Autodesk Inventor part; units mm, degrees
ref_plane "YZ Plane" through (0, 0, 0) normal (1, 0, 0) x (0, 1, 0)
ref_plane "XZ Plane" through (0, 0, 0) normal (0, 1, 0) x (-1, 0, 0)
ref_plane "XY Plane" through (0, 0, 0) normal (0, 0, 1) x (1, 0, 0)
sketch "Sketch1" plane through (0, 0, 0) normal (0, 0, 1) x (1, 0, 0)
  line L0 (37.0001, -37.0002) -> (-37.0001, -37.0002)
  line L1 (-37.0001, -37.0002) -> (-37.0001, 37.0002)
  line L2 (-37.0001, 37.0002) -> (37.0001, 37.0002)
  line L3 (37.0001, 37.0002) -> (37.0001, -37.0002)
  line L4 (69.0001, -5.0002) -> (-5.0001, 69.0002) construction
  circle A0 centre (32, 32) radius 1.5
  circle A1 centre (32, -32) radius 1.5
  circle A2 centre (-32, 32) radius 1.5
  line L5 (5.0001, -69.0002) -> (-69.0001, 5.0002) construction
  circle A3 centre (-32, -32) radius 1.5
  line L6 (37.0001, -101.0002) -> (-37.0001, -26.9998) construction
  line L7 (5.0001, -69.0002) -> (-69.0001, 5.0002) construction
extrude "Extrusion1" add sketch "Sketch1" along normal blind 22
fillet "Fillet1" radius 5 4 edges at (-37.0001, 37.0002, 11) (37.0001, 37.0002, 11) (37.0001, -37.0002, 11) (-37.0001, -37.0002, 11)
sketch "Sketch2" plane through (0, 0, 0) normal (0, 0, -1) x (-1, 0, 0)
  point P0 (0, 0)
sketch "Sketch4" plane through (0, 0, 22) normal (0, 0, 1) x (1, 0, 0)
  point P0 (0, 0)
sketch "Sketch5" plane through (0, 0, 22) normal (0, 0, 1) x (1, 0, 0)
  line L0 (-37.0001, 32.0002) -> (-37.0001, -32.0002)
  line L1 (-26.9999, 37.0018) -> (-37.0001, 37.0018)
  line L2 (-37.0001, 37.0018) -> (-37.0001, 26.9982)
  line L3 (-37.0001, 26.9982) -> (-26.9999, 26.9982)
  line L4 (-26.9999, 26.9982) -> (-26.9999, 37.0018)
  circle A0 centre (-32, 32) radius 1.5
  line L5 (-26.9999, 37.0018) -> (-37.0001, 26.9982) construction
  line L6 (-37.0001, 37.0018) -> (-26.9999, 26.9982) construction
  line L7 (37.0001, 37.0018) -> (26.9999, 37.0018)
  line L8 (26.9999, 37.0018) -> (26.9999, 26.9982)
  line L9 (26.9999, 26.9982) -> (37.0001, 26.9982)
  line L10 (37.0001, 26.9982) -> (37.0001, 37.0018)
  line L11 (37.0001, 37.0018) -> (26.9999, 26.9982) construction
  line L12 (26.9999, 37.0018) -> (37.0001, 26.9982) construction
  line L13 (-26.9999, -26.9982) -> (-37.0001, -26.9982)
  line L14 (-37.0001, -26.9982) -> (-37.0001, -37.0018)
  line L15 (-37.0001, -37.0018) -> (-26.9999, -37.0018)
  line L16 (-26.9999, -37.0018) -> (-26.9999, -26.9982)
  line L17 (-26.9999, -26.9982) -> (-37.0001, -37.0018) construction
  line L18 (-37.0001, -26.9982) -> (-26.9999, -37.0018) construction
  line L19 (37.0001, -26.9982) -> (26.9999, -37.0018) construction
  line L20 (37.0001, -37.0018) -> (37.0001, -26.9982)
  line L21 (26.9999, -37.0018) -> (37.0001, -37.0018)
  line L22 (26.9999, -26.9982) -> (26.9999, -37.0018)
  line L23 (37.0001, -26.9982) -> (26.9999, -26.9982)
  line L24 (26.9999, -26.9982) -> (37.0001, -37.0018) construction
  point P0 (0, 0)
extrude "Extrusion2" cut sketch "Sketch5" against normal blind 5 contours L2 L1 L4 L3 L0 | L13 L16 L15 L14 L0 | A0 | L10 L9 L8 L7 | L21 L22 L23 L20
fillet "Fillet2" radius 5 4 edges at (-26.9999, 26.9982, 19.5) (26.9999, 26.9982, 19.5) (-26.9999, -26.9982, 19.5) (26.9999, -26.9982, 19.5)
sketch "Sketch6" plane through (0, 0, 22) normal (0, 0, 1) x (1, 0, 0)
  line L0 (96.2626, 67.9332) -> (202.4541, 67.9332) construction
  line L1 (202.4541, 67.9332) -> (202.4541, -70.892) construction
  line L2 (202.4541, -70.892) -> (96.2626, -70.892) construction
  line L3 (96.2626, -70.892) -> (96.2626, 67.9332) construction
  point P0 (0, 0)
decal "Decal3"
properties part number "RTK-F9P-Sirius_rover"
The listing builds one solid part. Answer for the finished solid, in the listing's coordinates (mm). A direction names the side the tool comes from. Give positions to 0.01 mm unless a question says otherwise; leave off trailing zeros. Write each loop counter-clockwise with the first axis right and the second up, starting at its lowest first coordinate (ties: lowest second). Pieces come first, ordered by that corner, then holes.
Item 1: Section A-A, the plane z = 20 is taken. Write down the section's boundary in (x, y), plus the area to 3 significant figures.
Item 2: Determine the mould class of faces 1 (the cylindrical face through (-35, 36, 9)), 2 (the flat face through (-33.2, 33.2, 17)), 3 (the cylindrical face through (-33.2, 32.9, 8.4)) for opening direction X: released by +X, released by -X, zero draft, split by the parting line, or undercut.
Item 3: Find the intervals of material crossed by line 1 along Y through (x, z) = (32, 7); line 2 along X through (y, z) = (-32.5, 8.25), in increasing order.
Item 4: Flat-ended cylindrical pins translate along their axes: P1, Ø1.5, axis at y = -34, z = 20, coming from the +X side; P2, Ø5.5, axis at x = 34.5, z = 19, coming from the -Y side; P3, Ø2.5, axis at x = 33.5, z = 19, coming from the +Y side; P4, Ø1.8, axis at x = -32, y = 32, coming from the -Z side. Find the tip coordinate at first contact, or state that the pin passes through.
Item 5: Which of the six approach directions +Z, -Z, +X, -X, +Y, -Y give full straight-line access (tool end or side, diameter ignored) to faces 4 (the flat face through (-35, 26.998, 20)), 5 (the cylindrical face through (30.5, 31.93, 8.38)), 6 (the flat face through (-33.2, -30.8, 17)), 7 (the flat face through (27, -34, 20)), 8 (the flat face through (30.8, 33.2, 17))?
Completed:
1. outline: (-37, -27) - (-32, -27) arc R5 cw to (-27, -32) - (-27, -37) - (27, -37) - (27, -32) arc R5 cw to (32, -27) - (37, -27) - (37, 27) - (32, 27) arc R5 cw to (27, 32) - (27, 37) - (-27, 37) - (-27, 32) arc R5 cw to (-32, 27) - (-37, 27) - close
1. area: 5,100 mm2
2. face 1: released by -X
2. face 2: zero draft
2. face 3: undercut
3. line 1: y = -37 to -33.5, -30.5 to 30.5, 33.5 to 37
3. line 2: x = -36.98 to -33.41, -30.59 to 30.59, 33.41 to 36.98
4. P1: stops at x = 27
4. P2: stops at y = -36.96
4. P3: stops at y = 27
4. P4: passes through
5. face 4: +Z, -X, +Y
5. face 5: +Z, -Z
5. face 6: +Z, -X, -Y
5. face 7: +Z, +X, -Y
5. face 8: +Z, +X, +Y
